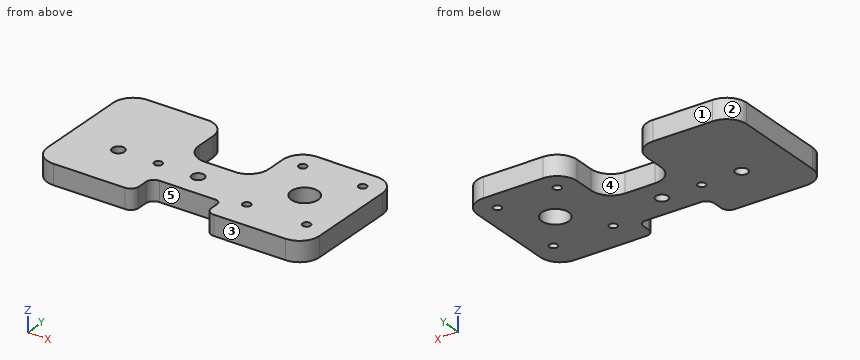
from build123d import *

# Parameters (mm, degrees)
MODEL_R             = 2
MODEL_R_2           = 3.05
MODEL_R_3           = 6.75
BOSS_EXTRUDE1_DEPTH = 10


with BuildPart() as part:
    # Model → Boss-Extrude1 (new body)
    with BuildSketch(Plane.XY):
        with BuildLine():
            Line((106.910569106, -1), (106.910569106, 3))
            ThreePointArc((106.910569106, 3), (106.031889449, 5.121320344), (103.910569106, 6))
            Line((103.910569106, 6), (75.910569106, 6))
            ThreePointArc((75.910569106, 6), (73.082141981, 4.828427125), (71.910569106, 2))
            Line((71.910569106, 2), (71.910569106, -3.03491552))
            ThreePointArc((71.910569106, -3.03491552), (70.73899623, -5.863342645), (67.910569106, -7.034915521))
            Line((67.910569106, -7.034915521), (31.910569106, -7.034915521))
            ThreePointArc((31.910569106, -7.034915521), (24.839501294, -4.105983332), (21.910569106, 2.96508448))
            Line((21.910569106, 2.96508448), (21.910569106, 50))
            ThreePointArc((21.910569106, 50), (24.839501294, 57.071067812), (31.910569106, 60))
            Line((31.910569106, 60), (61.910569106, 60))
            ThreePointArc((61.910569106, 60), (68.981636918, 57.071067812), (71.910569106, 50))
            Line((71.910569106, 50), (71.910569106, 40))
            ThreePointArc((71.910569106, 40), (74.839501294, 32.928932188), (81.910569106, 30))
            Line((81.910569106, 30), (96.910569106, 30))
            ThreePointArc((96.910569106, 30), (103.981636918, 32.928932188), (106.910569106, 40))
            Line((106.910569106, 40), (106.910569106, 50))
            ThreePointArc((106.910569106, 50), (109.839501294, 57.071067812), (116.910569106, 60))
            Line((116.910569106, 60), (146.910569106, 60))
            ThreePointArc((146.910569106, 60), (153.981636918, 57.071067812), (156.910569106, 50))
            Line((156.910569106, 50), (156.910569106, 5))
            ThreePointArc((156.910569106, 5), (153.981636918, -2.071067812), (146.910569106, -5))
            Line((146.910569106, -5), (110.910569106, -5))
            ThreePointArc((110.910569106, -5), (108.082141981, -3.828427125), (106.910569106, -1))
        make_face()
        with Locations((66.910569106, 18)):
            Circle(MODEL_R, mode=Mode.SUBTRACT)
        with Locations((46.910569106, 18)):
            Circle(MODEL_R_2, mode=Mode.SUBTRACT)
        with Locations((116.910569106, 10)):
            Circle(MODEL_R, mode=Mode.SUBTRACT)
        with Locations((146.910569106, 10)):
            Circle(MODEL_R, mode=Mode.SUBTRACT)
        with Locations((146.910569106, 50)):
            Circle(MODEL_R, mode=Mode.SUBTRACT)
        with Locations((116.910569106, 50)):
            Circle(MODEL_R, mode=Mode.SUBTRACT)
        with Locations((131.910569106, 30)):
            Circle(MODEL_R_3, mode=Mode.SUBTRACT)
        with Locations((86.910569106, 18)):
            Circle(MODEL_R_2, mode=Mode.SUBTRACT)
    extrude(amount=BOSS_EXTRUDE1_DEPTH)


solid = part.part
Geometry: final body of the model. Coordinates: model frame, mm. Face numbers are marked on the shaded views. A direction names the side the tool comes from. Coordinates: 2 decimals unless noted, no trailing zeros. Order: outer loops, then holes, each group sorted by start corner. A loop starts at its lowest first (then second) coordinate and runs counter-clockwise, first axis right, second up. Notation, with made-up numbers: (65.5, 27.25) - (78.5, 27.25) arc R20 ccw to (78.5, 45.25) - close; hole circle Ø11 at (75, 64). An arc over 180 degrees is marked (long way). Use one line per item in the form item = value.
1) Section A-A (y = 10). Return loops of the section in (x, z), then the cut area to 3 significant figures.
Solutions:
outline = (21.91, 0) - (114.91, 0) - (114.91, 10) - (21.91, 10) - close; (118.91, 0) - (144.91, 0) - (144.91, 10) - (118.91, 10) - close; (148.91, 0) - (156.91, 0) - (156.91, 10) - (148.91, 10) - close
area = 1,270 mm^2
2) Section D-D (y = 0.5). Return loops of the section in (x, z).
Solutions:
outline = (22.22, 0) - (71.91, 0) - (71.91, 10) - (22.22, 10) - close; (106.91, 0) - (155.84, 0) - (155.84, 10) - (106.91, 10) - close
3) Ray query, L1, parallel to Y at x = 82, z = 4.25; L2, parallel to X at y = 54, z = 8; L3, parallel to Y at x = 129, z = 8.75. Return the intervals inside material, ascending.
Solutions:
L1 = 6 to 30
L2 = 22.75 to 71.08, 107.75 to 156.08
L3 = -5 to 23.91, 36.09 to 60
4) Section B-B (y = 18). Return loops of the section in (x, z), then the cut area to 3 significant figures.
Solutions:
outline = (21.91, 0) - (43.86, 0) - (43.86, 10) - (21.91, 10) - close; (49.96, 0) - (64.91, 0) - (64.91, 10) - (49.96, 10) - close; (68.91, 0) - (83.86, 0) - (83.86, 10) - (68.91, 10) - close; (89.96, 0) - (156.91, 0) - (156.91, 10) - (89.96, 10) - close
area = 1,190 mm^2
5) Set-up query: the marked faces 1, 2, 3, 4 and 5. Return all of +Z, -Z, +X, -X, +Y, -Y with unobstructed straight access to the full face (end or side cutting, diameter ignored); none if empty.
Solutions:
face_1 = +Z, -Z, +X, -X, +Y
face_2 = +Z, -Z, -X, +Y
face_3 = +Z, -Z, +X, -Y
face_4 = +Z, -Z, +Y
face_5 = +Z, -Z, -Y
6) Pin query (flat end, axial travel): pin 1 (2.5 mm diameter, centred on x = 116.91, y = 50, fed in from +Z); pin 2 (1 mm diameter, centred on x = 98.5, z = 5, fed in from -Y); pin 3 (3 mm diameter, centred on x = 128.5, z = 5.5, fed in from -Y); pin 4 (5.5 mm diameter, centred on y = 0, z = 5.5, fed in from +X). Return the tip coordinate at first contact, or that it passes through.
Solutions:
pin_1 = through
pin_2 = 6
pin_3 = -5
pin_4 = 156.65
7) Section C-C (z = 5). State how many separate pieces and enclosed holes the cut face has, then the cut area to 3 significant figures.
Solutions:
separate_pieces = 1
enclosed_holes = 8
area = 7,090 mm^2
